```python
from build123d import *

# Parameters (mm, degrees)
F0_R     = 231
F0_R_2   = 229
F1_DEPTH = 30
F2_W     = 30
F2_H     = 30
F3_DEPTH = 3
F4_R     = 4
F5_DEPTH = 25
F6_R     = 10
F8_COUNT = 4
F9_SIZE  = 2.99999


# Not quite as in the source:
# - a fillet or chamfer is up to 0.001 mm smaller than in the source, because OpenCascade refuses the exact size


with BuildPart() as f1:
    # F0 (on Top) → F1 (new body)
    with BuildSketch(Plane.XY):
        Circle(F0_R)
        Circle(F0_R_2, mode=Mode.SUBTRACT)
    extrude(amount=F1_DEPTH)

    # F2 (on face) → F3 (join)
    with BuildSketch(Plane(origin=(0, 0, 0), x_dir=(1, 0, 0), z_dir=(0, 0, -1))):
        with Locations((0, -245.5124725476)):
            Rectangle(F2_W, F2_H)
    extrude(amount=-F3_DEPTH)

    # F4 (on face) → F5 (cut)
    with BuildSketch(Plane(origin=(0, 0, 0), x_dir=(1, 0, 0), z_dir=(0, 0, -1))):
        with Locations((0, -245.5124725476)):
            Circle(F4_R)
    extrude(amount=-F5_DEPTH, mode=Mode.SUBTRACT)

    # F6
    f6_edges = [f1.edges().sort_by_distance(p)[0] for p in [
        (-15, 260.512473, 1.5),
        (15, 260.512473, 1.5),
    ]]
    fillet(f6_edges, radius=F6_R)

    # F8: F1 ×4 about axis
    f8_axis = Axis((0, 0, -51.1162020266), (0, 0, -1))


with BuildPart() as f1_1:
    add(f1.part)
    for i in range(1, F8_COUNT):
        add(f1.part.rotate(f8_axis, i * 360 / F8_COUNT))

    # F9 (size 3 in the source; OpenCascade refuses exactly that, so slightly less here)
    f9_edges = [f1_1.edges().sort_by_distance(p)[0] for p in [
        (-245.512473, -4, 3),
        (-4, 245.512473, 3),
        (245.512473, 4, 3),
        (4, -245.512473, 3),
    ]]
    chamfer(f9_edges, length=F9_SIZE)


solid = f1_1.part
```
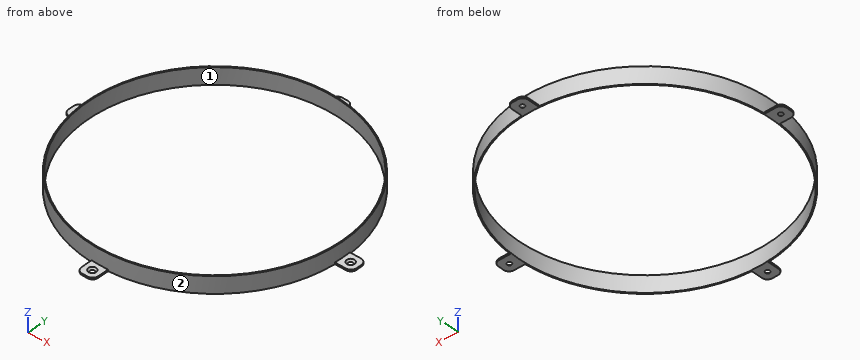
Check sheet for the modelled part. Datum: model origin and axes. Units: mm. Face numbers are marked on the shaded views. Round coordinates to 2 decimals unless told otherwise and drop trailing zeros. Order: outer loops, then holes, each group sorted by start corner. A loop starts at its lowest first (then second) coordinate and runs counter-clockwise, first axis right, second up. Notation, with made-up numbers: (78, 41) -> (87, 41) arc R28 ccw to (87, 62) -> close; hole circle Ø4 at (64.25, 37.25). An arc over 180 degrees is marked (long way). Use CSV: the item, a comma, the result in double quotes.
(1) Depth check by flat-ended pin: pin 1 (3.5 mm diameter, centred on y = 241, z = 2, fed in from +X); pin 2 (15 mm diameter, centred on x = 3, y = 246, fed in from +Z); pin 3 (6 mm diameter, centred on x = 76, z = 19, fed in from -Y). Enter the tip coordinate at first touch or a pass-through.
Worked out:
pin 1,"x = 15"
pin 2,"z = 3"
pin 3,"y = -219.16"
(2) Cross-section at A-A (y = 53.5). Record the boundary of the cut face in (x, z).
Worked out:
outline,"(-224.72, 0) -> (-222.66, 0) -> (-222.66, 30) -> (-224.72, 30) -> close; (222.66, 0) -> (224.72, 0) -> (224.72, 30) -> (222.66, 30) -> close"
(3) Cross-section at B-B (x = 122). Record the boundary of the cut face in (y, z).
Worked out:
outline,"(-196.16, 0) -> (-193.8, 0) -> (-193.8, 30) -> (-196.16, 30) -> close; (193.8, 0) -> (196.16, 0) -> (196.16, 30) -> (193.8, 30) -> close"
(4) Draft check along Y on the marked faces 1 and 2. Enter one of: pulls with the +Y half, pulls with the -Y half, needs draft (parallel to the pull), parting line crosses it, or undercut.
Worked out:
face 1,"undercut"
face 2,"parting line crosses it"
(5) Cross-section at C-C (z = 9.25). Record the boundary of the cut face in (x, y).
Worked out:
outline,"circle Ø462 at (0, 0); hole circle Ø458 at (0, 0)"
(6) Material ranges on line 1 along Y through (x, z) = (0, 0.05); line 2 along X through (y, z) = (5.5, 24.5); line 3 along X through (y, z) = (0, 11.5), recorded low to high. Write a range as from..to.
Worked out:
line 1,"-260.51..-249.56, -241.46..-229, 229..241.46, 249.56..260.51"
line 2,"-230.93..-228.93, 228.93..230.93"
line 3,"-231..-229, 229..231"
